The listing builds one solid part. Answer for the finished solid, in the listing's coordinates (mm). A direction names the side the tool comes from. Coordinates: 2 decimals unless noted, no trailing zeros. Order: outer loops, then holes, each group sorted by start corner. A loop starts at its lowest first (then second) coordinate and runs counter-clockwise, first axis right, second up. Notation, with made-up numbers: M -9,-18 L 43,-18 A18 ccw 43,0 Z; hole C 44,21.5 d11. An arc over 180 degrees is marked long. One line per item, written item: value. Start each with the question number.
Q1. The part is cut by section C-C on z = 0.5. Give the number of separate pieces and of enclosed holes in the cut face, then the cut area to 3 significant figures.
Q2. Straight lines are drawn through the part: line 1 along Z through (x, y) = (-20, -11.3); line 2 along Y through (x, z) = (-27.25, 0); line 3 along Y through (x, z) = (-42.55, 0). For each, find the intervals that lie inside material, in ascending order. Write a range as [from, to].
Q3. The part is cut by section D-D on x = -34. Give the vertices of the cut face in (y, z), then the cut area to 3 significant figures.
Q4. The part is cut by section A-A on x = -48. Give the vertices of the cut face in (y, z), then the cut area to 3 significant figures.
Q5. For faces 1 (the flat face through (-18.6, -9, 1.2)), 2 (the cylindrical face through (-34, -8, -2)), 3 (the flat face through (-32.75, 12, 0)), 4 (the cylindrical face through (-38.58, 8.44, -0.35)), determine the directions among +Z, -Z, +X, -X, +Y, -Y from which every point of the face is accessible in a straight line to the end or side of a thin tool.
Q6. Determine the mould class of faces 5 (the cylindrical face through (-46.474, -11.535, -0.481)), 6 (the cylindrical face through (-34, -7, 3)), 7 (the flat face through (-34, -14, 0)), 8 (the flat face through (-23, 3, 0)) for opening direction X: pulls with the +X half, pulls with the -X half, needs draft (parallel to the pull), parting line crosses it, or undercut.
Q7. Each of these flat-tipped pins is pushed along its axis until it touches: pin 1 Ø1.5 at (y, z) = (-2, 2) entering from +X; pin 2 Ø4 at (x, z) = (-48, 0) entering from +Y; pin 3 Ø3 at (y, z) = (9, 0.5) entering from -X. Where does it stop, or does it pass through?
Q8. The part is cut by section B-B on y = 10. Give the vertices of the cut face in (x, z), then the cut area to 3 significant figures.
```python
from build123d import *

# Parameters (mm, degrees)
SKETCH1_W                      = 22
SKETCH1_H                      = 29
BOSS_EXTRUDE1_DEPTH            = 5
SKETCH3_W                      = 34
SKETCH3_H                      = 10
BOSS_EXTRUDE2_DEPTH            = 5
F_16_0_16_DIAMETER_HOLE1_D     = 16
F_16_0_16_DIAMETER_HOLE1_DEPTH = 6
F_14_0_14_DIAMETER_HOLE1_D     = 14
M3_CLEARANCE_HOLE1_D           = 3.2
SKETCH12_W                     = 2.5
SKETCH12_H                     = 8.112511343
CUT_EXTRUDE1_DEPTH             = 25.779023387
CBORE_FOR_M3_SHCS1_D           = 3.2
CBORE_FOR_M3_SHCS1_DEPTH       = 9.75
CBORE_FOR_M3_SHCS1_CBORE_D     = 6.5
CBORE_FOR_M3_SHCS1_CBORE_DEPTH = 3
CHAMFER1_SIZE                  = 0.5
M3X0_5_TAPPED_HOLE1_D          = 2.5


with BuildPart() as part:
    # Sketch1 → Boss-Extrude1 (new, symmetric)
    with BuildSketch(Plane.XY):
        with Locations((0, 0.5)):
            Rectangle(SKETCH1_W, SKETCH1_H)
    extrude(amount=BOSS_EXTRUDE1_DEPTH, both=True)

    # Sketch3 → Boss-Extrude2 (add)
    with BuildSketch(Plane.XZ.offset(14)):
        Rectangle(SKETCH3_W, SKETCH3_H)
    extrude(amount=-BOSS_EXTRUDE2_DEPTH)

    # Ø16.0 (16) Diameter Hole1
    with Locations(Plane(origin=(0, 0, -5), x_dir=(-1, 0, 0), z_dir=(0, 0, -1))):
        with Locations((0, 0)):
            Hole(F_16_0_16_DIAMETER_HOLE1_D / 2, depth=F_16_0_16_DIAMETER_HOLE1_DEPTH)

    # Ø14.0 (14) Diameter Hole1 (through all)
    with Locations(Plane(origin=(0, 0, 1), x_dir=(-1, 0, 0), z_dir=(0, 0, -1))):
        with Locations((0, 0)):
            Hole(F_14_0_14_DIAMETER_HOLE1_D / 2)

    # M3 Clearance Hole1 (through all)
    with Locations(Plane(origin=(0, -9, 0), x_dir=(1, 0, 0), z_dir=(0, 1, 0))):
        with Locations((-14, 0), (14, 0)):
            Hole(M3_CLEARANCE_HOLE1_D / 2)

    # Sketch12 → Cut-Extrude1 (cut, through all)
    with BuildSketch(Plane.XY.offset(5)):
        with Locations((0, 10.943744329)):
            Rectangle(SKETCH12_W, SKETCH12_H)
    extrude(amount=-CUT_EXTRUDE1_DEPTH, mode=Mode.SUBTRACT)

    # CBORE for M3 SHCS1
    with Locations(Plane(origin=(11, 0, 0), x_dir=(0, 0, -1), z_dir=(1, 0, 0))):
        with Locations((0, 10)):
            CounterBoreHole(CBORE_FOR_M3_SHCS1_D / 2, CBORE_FOR_M3_SHCS1_CBORE_D / 2, CBORE_FOR_M3_SHCS1_CBORE_DEPTH, depth=CBORE_FOR_M3_SHCS1_DEPTH)

    # Chamfer1
    chamfer1_edges = [part.edges().sort_by_distance(p)[0] for p in [
        (0, -8, -5),
    ]]
    chamfer(chamfer1_edges, length=CHAMFER1_SIZE)


with BuildPart() as body_2:
    # Mirror1: mirrored copy
    add(part.part.mirror(Plane(origin=(-17, -9, -5), x_dir=(0, 0, 1), z_dir=(-1, 0, 0))))

    # M3x0.5 Tapped Hole1 (through all)
    with Locations(Plane(origin=(-23, 0, 0), x_dir=(0, 0, -1), z_dir=(1, 0, 0))):
        with Locations((0, 10)):
            Hole(M3X0_5_TAPPED_HOLE1_D / 2)


solid = body_2.part
```
Output:
1. separate pieces: 5
1. enclosed holes: 0
1. area: 387 mm^2
2. line 1: z = [-5, -1.6], [1.6, 5]
2. line 2: y = [-14, -4.29], [4.29, 8.75], [11.25, 15]
2. line 3: y = [-14, 6.75], [13.25, 15]
3. outline: M -14,-5 L -8.5,-5 L -8,-4.5 L -8,1 L -7,1 L -7,5 L -14,5 Z
3. area: 63.9 mm^2
4. outline: M -14,-5 L -9,-5 L -9,-1.6 L -14,-1.6 Z; M -14,1.6 L -9,1.6 L -9,5 L -14,5 Z
4. area: 34.0 mm^2
5. face 1: +Z, -Z, +X, +Y
5. face 2: -Z
5. face 3: +Z, -Z, +Y
5. face 4: -X
6. face 5: undercut
6. face 6: undercut
6. face 7: needs draft
6. face 8: pulls with the +X half
7. pin 1: stops at x = -23
7. pin 2: stops at y = -9
7. pin 3: stops at x = -42
8. outline: M -45,-5 L -35.25,-5 L -35.25,-1.6 L -42,-1.6 L -42,-3.25 L -45,-3.25 Z; M -45,3.25 L -42,3.25 L -42,1.6 L -35.25,1.6 L -35.25,5 L -45,5 Z; M -32.75,-5 L -23,-5 L -23,-1.25 L -32.75,-1.25 Z; M -32.75,1.25 L -23,1.25 L -23,5 L -32.75,5 Z
8. area: 130 mm^2
